Verification items for the finished model (mm, model axes). A direction names the side the tool comes from. Give positions to 0.01 mm unless a question says otherwise; leave off trailing zeros. Loops run counter-clockwise (first coordinate to the right, second up) from the corner with the lowest first, then second, coordinate; pieces in that order, holes last. Notation, with made-up numbers: M 50.25,27 L 58.25,27 A24 cw 58.25,37 Z; hole C 25.5,12.25 d3. An arc over 180 degrees is marked long. Answer in a Markdown table with one row per item.
```python
from build123d import *

# Parameters (mm, degrees)
F1_DEPTH = 3
F2_DEPTH = 5


with BuildPart() as f1:
    # F0 (on Front) → F1 (new body)
    with BuildSketch(Plane.XZ):
        with BuildLine():
            Line((-23, 0), (-8, 0))
            ThreePointArc((-8, 0), (-2.3431457505, 2.3431457505), (0, 8))
            Line((0, 8), (0, 15))
            ThreePointArc((0, 15), (-2.3431457505, 20.6568542495), (-8, 23))
            Line((-8, 23), (-23, 23))
            ThreePointArc((-23, 23), (-28.6568542495, 20.6568542495), (-31, 15))
            Line((-31, 15), (-31, 8))
            ThreePointArc((-31, 8), (-28.6568542495, 2.3431457505), (-23, 0))
        make_face()
        with BuildLine():
            add(Edge.make_bspline(
                [(-26.3173828125, 12.5717230903), (-25.6740451389, 11.8448350694), (-25.6740451389, 10.6067708333)],
                knots=[0, 0, 0, 1, 1, 1], degree=2))
            add(Edge.make_bspline(
                [(-25.6740451389, 10.6067708333), (-25.6740451389, 9.3337673611), (-26.3143446181, 8.6190321181)],
                knots=[0, 0, 0, 1, 1, 1], degree=2))
            add(Edge.make_bspline(
                [(-26.3143446181, 8.6190321181), (-26.9546440972, 7.904296875), (-28.0848524306, 7.904296875)],
                knots=[0, 0, 0, 1, 1, 1], degree=2))
            add(Edge.make_bspline(
                [(-28.0848524306, 7.904296875), (-28.7836371528, 7.904296875), (-29.3244357639, 8.232421875)],
                knots=[0, 0, 0, 1, 1, 1], degree=2))
            add(Edge.make_bspline(
                [(-29.3244357639, 8.232421875), (-29.865234375, 8.560546875), (-30.1599392361, 9.1727430556)],
                knots=[0, 0, 0, 1, 1, 1], degree=2))
            add(Edge.make_bspline(
                [(-30.1599392361, 9.1727430556), (-30.4546440972, 9.7849392361), (-30.4546440972, 10.6067708333)],
                knots=[0, 0, 0, 1, 1, 1], degree=2))
            add(Edge.make_bspline(
                [(-30.4546440972, 10.6067708333), (-30.4546440972, 11.8782552083), (-29.8181423611, 12.5884331597)],
                knots=[0, 0, 0, 1, 1, 1], degree=2))
            add(Edge.make_bspline(
                [(-29.8181423611, 12.5884331597), (-29.181640625, 13.2986111111), (-28.0514322917, 13.2986111111)],
                knots=[0, 0, 0, 1, 1, 1], degree=2))
            add(Edge.make_bspline(
                [(-28.0514322917, 13.2986111111), (-26.9607204861, 13.2986111111), (-26.3173828125, 12.5717230903)],
                knots=[0, 0, 0, 1, 1, 1], degree=2))
        make_face(mode=Mode.SUBTRACT)
        Polygon((-20.1579996961, 8.4896369224), (-20.1579996961, 3.7006579805), (-21.4600723116, 3.7006579805), (-21.4600723116, 14.904367548), (-15.2145375625, 14.904367548), (-15.2145375625, 13.7469696675), (-20.1579996961, 13.7469696675), (-20.1579996961, 9.6470348028), (-15.5136954893, 9.6470348028), (-15.5136954893, 8.4896369224), align=None, mode=Mode.SUBTRACT)
        Polygon((-4.8543552639, 14.904367548), (-4.8543552639, 3.7006579805), (-6.1564278794, 3.7006579805), (-6.1564278794, 8.9727034106), (-12.0586666469, 8.9727034106), (-12.0586666469, 3.7006579805), (-13.3607392625, 3.7006579805), (-13.3607392625, 14.904367548), (-12.0586666469, 14.904367548), (-12.0586666469, 10.1374576335), (-6.1564278794, 10.1374576335), (-6.1564278794, 14.904367548), align=None, mode=Mode.SUBTRACT)
    extrude(amount=F1_DEPTH)

    # F0 (on Front) → F2 (join)
    with BuildSketch(Plane.XZ):
        with BuildLine():
            Line((-0.4425173427, 31.5346689522), (-30.4425173427, 31.5346689522))
            ThreePointArc((-30.4425173427, 31.5346689522), (-33.9780512487, 30.0702028582), (-35.4425173427, 26.5346689522))
            Line((-35.4425173427, 26.5346689522), (-35.4425173427, -3.4653310478))
            ThreePointArc((-35.4425173427, -3.4653310478), (-33.9780512487, -7.0008649537), (-30.4425173427, -8.4653310478))
            Line((-30.4425173427, -8.4653310478), (-0.4425173427, -8.4653310478))
            ThreePointArc((-0.4425173427, -8.4653310478), (3.0930165632, -7.0008649537), (4.5574826573, -3.4653310478))
            Line((4.5574826573, -3.4653310478), (4.5574826573, 26.5346689522))
            ThreePointArc((4.5574826573, 26.5346689522), (3.0930165632, 30.0702028582), (-0.4425173427, 31.5346689522))
        make_face()
        with BuildLine():
            ThreePointArc((0, 8), (-2.3431457505, 2.3431457505), (-8, 0))
            Line((-8, 0), (-23, 0))
            ThreePointArc((-23, 0), (-28.6568542495, 2.3431457505), (-31, 8))
            Line((-31, 8), (-31, 15))
            ThreePointArc((-31, 15), (-28.6568542495, 20.6568542495), (-23, 23))
            Line((-23, 23), (-8, 23))
            ThreePointArc((-8, 23), (-2.3431457505, 20.6568542495), (0, 15))
            Line((0, 15), (0, 8))
        make_face(mode=Mode.SUBTRACT)
    extrude(amount=F2_DEPTH)


solid = f1.part
```
Item 1: Sectioned sample at C-C (y = -4.05). Record the cut outline in (x, z).
Reported:
| item | result |
|---|---|
| outline | M -35.44,-3.47 A5 ccw -30.44,-8.47 L -0.44,-8.47 A5 ccw 4.56,-3.47 L 4.56,26.53 A5 ccw -0.44,31.53 L -30.44,31.53 A5 ccw -35.44,26.53 Z; hole M -31,8 A8 ccw -23,0 L -8,0 A8 ccw 0,8 L 0,15 A8 ccw -8,23 L -23,23 A8 ccw -31,15 Z |
Item 2: Sectioned sample at D-D (z = 6.5). Record the cut outline in (x, y), and give its area (3 significant figures).
Reported:
| item | result |
|---|---|
| outline | M -35.44,-5 L -30.86,-5 L -30.86,-3 L -21.46,-3 L -21.46,0 L -35.44,0 Z; M -20.16,-3 L -13.36,-3 L -13.36,0 L -20.16,0 Z; M -12.06,-3 L -6.16,-3 L -6.16,0 L -12.06,0 Z; M -4.85,-3 L -0.14,-3 L -0.14,-5 L 4.56,-5 L 4.56,0 L -4.85,0 Z |
| area | 127 mm^2 |
Item 3: Scan lines: L1, parallel to Z at x = -12, y = -0.7; L2, parallel to X at y = -4.2, z = 14; L3, parallel to Z at x = -10, y = -4.3. Record each from-to range of solid material in increasing order. Write a range as [from, to].
Reported:
| item | result |
|---|---|
| L1 | z = [-8.47, 8.97], [10.14, 31.53] |
| L2 | x = [-35.44, -31], [0, 4.56] |
| L3 | z = [-8.47, 0], [23, 31.53] |
Item 4: Tool access check on faces 1 (the flat face through (-9, -1, 10.137)), 2 (the flat face through (-15, -2, 31.535)), 3 (the cylindrical face through (-2.406, -3.986, 20.719)). Record the directions out of +Z, -Z, +X, -X, +Y, -Y that give a thin tool (end or side, any length) a straight path to the whole face; none if there is none.
Reported:
| item | result |
|---|---|
| face 1 | +Y, -Y |
| face 2 | +Z, +X, -X, +Y, -Y |
| face 3 | -Y |
Item 5: Release check for a two-part mould opening along X. For faces 4 (the cylindrical face through (-2.281, -3.986, 2.406)), 5 (the flat face through (-35.443, -2, 12)), 6 (the cylindrical face through (3.13, -2.46, 30.03)) record: released by +X, released by -X, zero draft, split by the parting line, or undercut.
Reported:
| item | result |
|---|---|
| face 4 | undercut |
| face 5 | released by -X |
| face 6 | released by +X |
Item 6: Go/stop test with a flat-tipped pin: pin 1 (10 mm diameter, centred on x = -10, z = 16, fed in from -Y). Record where the tip stops, or that it passes through.
Reported:
| item | result |
|---|---|
| pin 1 | stops at y = -3 |
Item 7: Sectioned sample at B-B (x = -17). Record the cut outline in (y, z), and give its area (3 significant figures).
Reported:
| item | result |
|---|---|
| outline | M -5,-8.47 L 0,-8.47 L 0,8.49 L -3,8.49 L -3,0 L -5,0 Z; M -5,23 L -3,23 L -3,14.9 L 0,14.9 L 0,31.53 L -5,31.53 Z; M -3,9.65 L 0,9.65 L 0,13.75 L -3,13.75 Z |
| area | 147 mm^2 |
Item 8: Sectioned sample at A-A (x = -9). Record the cut outline in (y, z).
Reported:
| item | result |
|---|---|
| outline | M -5,-8.47 L 0,-8.47 L 0,8.97 L -3,8.97 L -3,0 L -5,0 Z; M -5,23 L -3,23 L -3,10.14 L 0,10.14 L 0,31.53 L -5,31.53 Z |
